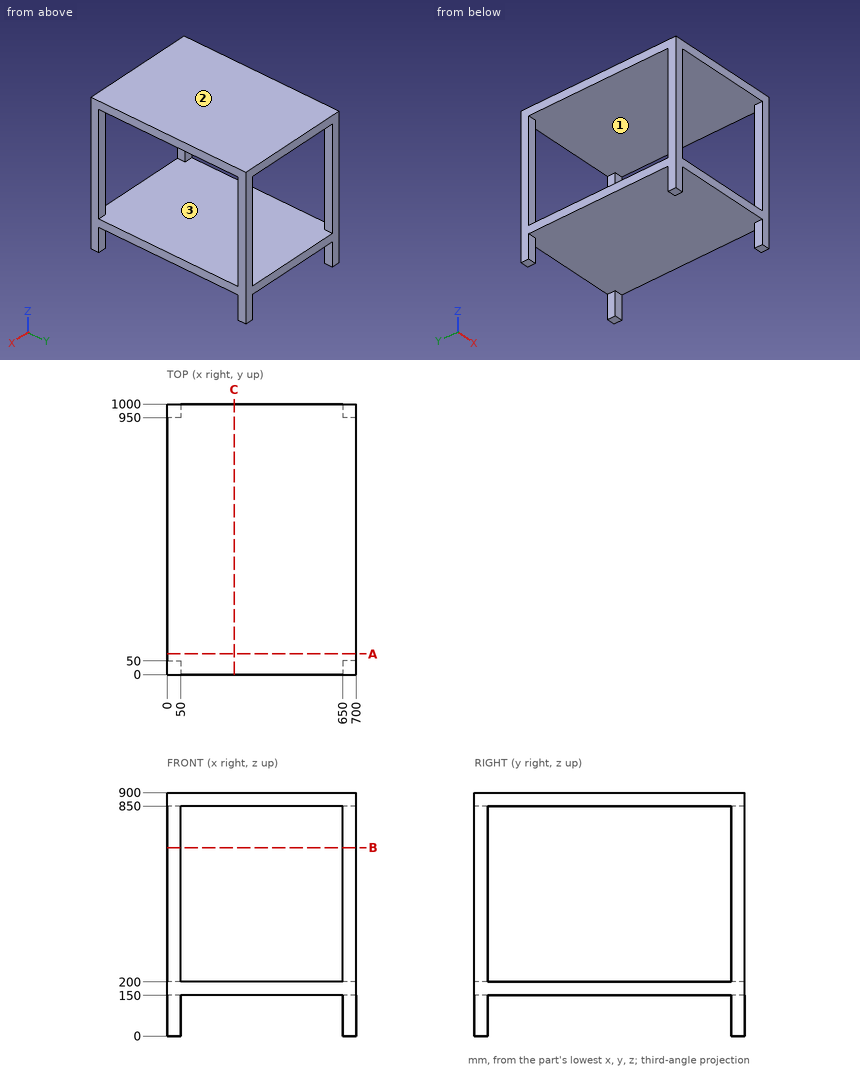
Drawing for the job (mm, zero at the part's lowest x, y, z). Round coordinates to 2 decimals unless told otherwise and drop trailing zeros. Loops run counter-clockwise (first coordinate to the right, second up) from the corner with the lowest first, then second, coordinate; pieces in that order, holes last. Notation, with made-up numbers: M -26,-35.75 L -14,-35.75 A27 cw -14,-16.75 Z; hole C 53.25,-10.5 d3. An arc over 180 degrees is marked long. Use a Markdown table: item, result. Add a question column.
(1) Cut at C-C (x = 248). Give the cut face in (y, z), and give its area (3 significant figures).
(2) Cut at A-A (y = 76.5). Give the cut face in (x, z).
(3) Pull direction Z, two halves, no side cores. Call the marked faces 1, 2 and 3: +Z half, -Z half, draft (parallel to the pull), parting line (faces both ways), or undercut.
(4) Cut at B-B (z = 696.5). Give the cut face in (x, y), and give its area (3 significant figures).
(5) Drill centre lines: line 1 (Z direction, x = 318.5, y = 683.5); line 2 (X direction, y = 958.5, z = 841). Where is each one in solid material? Low to high.
Geometry says:
| question | item | result |
|---|---|---|
| 1 | outline | M 0,150 L 1000,150 L 1000,200 L 0,200 Z; M 0,850 L 1000,850 L 1000,900 L 0,900 Z |
| 1 | area | 100,000 mm² |
| 2 | outline | M 0,150 L 700,150 L 700,200 L 0,200 Z; M 0,850 L 700,850 L 700,900 L 0,900 Z |
| 3 | face 1 | undercut |
| 3 | face 2 | +Z half |
| 3 | face 3 | undercut |
| 4 | outline | M 0,0 L 50,0 L 50,50 L 0,50 Z; M 0,950 L 50,950 L 50,1000 L 0,1000 Z; M 650,0 L 700,0 L 700,50 L 650,50 Z; M 650,950 L 700,950 L 700,1000 L 650,1000 Z |
| 4 | area | 10,000 mm² |
| 5 | line 1 | z = 150 to 200, 850 to 900 |
| 5 | line 2 | x = 0 to 50, 650 to 700 |
